Geometry: final body of the model. Coordinates: model frame, mm. Face numbers are marked on the shaded views. A direction names the side the tool comes from. Round coordinates to 2 decimals unless told otherwise and drop trailing zeros. Loops run counter-clockwise (first coordinate to the right, second up) from the corner with the lowest first, then second, coordinate; pieces in that order, holes last. Notation, with made-up numbers: M 0,-3.75 L 40,-3.75 A18 ccw 40,20.25 Z; hole C 5,-39.5 d3. An arc over 180 degrees is marked long. Answer as a JSON object with one key per item and string values.
from build123d import *

# Parameters (mm, degrees)
SKETCH_1_R          = 4.5
EXTRUDE_1_DEPTH     = 55
EXTRUDE_2_DEPTH     = 15
SKETCH_4_R          = 2
CUT_EXTRUDE_1_DEPTH = 71.544312315
CUT_EXTRUDE_3_DEPTH = 71.544312315
FILLET_1_R          = 0.5


with BuildPart() as part:
    # 草图1 → 凸台-拉伸1 (new body)
    with BuildSketch(Plane(origin=(0, 0, 0), x_dir=(1, 0, 0), z_dir=(0, 1, 0))):
        with Locations(Location((0, 0, 0), (0, 0, 270))):
            Circle(SKETCH_1_R)
    extrude(amount=EXTRUDE_1_DEPTH)

    # 草图2 → 凸台-拉伸2 (add)
    with BuildSketch(Plane(origin=(0, 55, 0), x_dir=(1, 0, 0), z_dir=(0, 1, 0))):
        with BuildLine():
            Line((-3, 3.010398645), (-3, -3.010398645))
            ThreePointArc((-3, -3.010398645), (0, -4.25), (3, -3.010398645))
            Line((3, -3.010398645), (3, 3.010398645))
            ThreePointArc((3, 3.010398645), (0, 4.25), (-3, 3.010398645))
        make_face()
    extrude(amount=EXTRUDE_2_DEPTH)

    # 草图4 → 切除-拉伸1 (cut, through all)
    with BuildSketch(Plane.ZY.offset(3)):
        with Locations((0, 61.5)):
            Circle(SKETCH_4_R)
    extrude(amount=-CUT_EXTRUDE_1_DEPTH, mode=Mode.SUBTRACT)

    # 草图5 → 切除-拉伸3 (cut, through all)
    with BuildSketch(Plane.ZY.offset(3)):
        with BuildLine():
            Line((-4.813255022, 64.251745482), (-4.813255022, 72.406434262))
            Line((-4.813255022, 72.406434262), (5.466876832, 72.406434262))
            Line((5.466876832, 72.406434262), (5.466876832, 63.634516306))
            ThreePointArc((5.466876832, 63.634516306), (0.449497866, 65.986517994), (-4.813255022, 64.251745482))
        make_face()
    extrude(amount=-CUT_EXTRUDE_3_DEPTH, mode=Mode.SUBTRACT)

    # 圆角1
    fillet_1_edges = [part.edges().sort_by_distance(p)[0] for p in [
        (0, 64.679603547, -4.25),
        (0, 64.679603547, 4.25),
    ]]
    fillet(fillet_1_edges, radius=FILLET_1_R)


solid = part.part
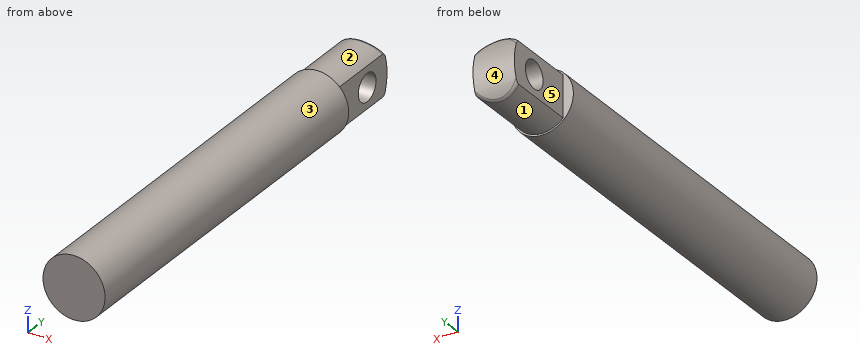
1) Ray query, line 1 (Y direction, x = -1.4, z = 0); line 2 (X direction, y = 60.5, z = -3.75); line 3 (X direction, y = 53, z = -2). Return the intervals inside material, ascending.
Results:
{"line 1": "0 to 59.5, 63.5 to 66", "line 2": "-2 to 2", "line 3": "-4.03 to 4.03"}
2) Section query A-A (z = 0). Return the cut outline in (x, y).
Results:
{"outline": "M -4.5,0 L 4.5,0 L 4.5,55 L 3,55 L 3,59.5 L -3,59.5 L -3,55 L -4.5,55 Z; M -3,63.5 L 3,63.5 L 3,66 L -3,66 Z"}
3) Reachability of the marked faces 1, 2, 3, 4 and 5 from +Z, -Z, +X, -X, +Y, -Y: full face, straight path, thin tool, end or side. Return the list, or none.
Results:
{"face 1": "-Z, +Y", "face 2": "+Z, +Y", "face 3": "+Y, -Y", "face 4": "+X, -X, +Y", "face 5": "+Z, -Z, -X, +Y"}
4) Section query C-C (y = 35.5). Return the cut outline in (x, z), and give its area (3 significant figures).
Results:
{"outline": "C 0,0 d9", "area": "63.6 mm2"}
5) Pin query (flat end, axial travel): P1, Ø5, axis at y = 61, z = 0.5, coming from the +X side; P2, Ø1, axis at y = 12, z = -1, coming from the +X side; P3, Ø4.5, axis at y = 61.5, z = 0, coming from the -X side; P4, Ø1.8, axis at y = 62, z = 0, coming from the -X side. Return the tip coordinate at first contact, or that it passes through.
Results:
{"P1": "x = 3", "P2": "x = 4.47", "P3": "x = -3", "P4": "through"}
6) Section query B-B (y = 61.5). Return the cut outline in (x, z), and give its area (3 significant figures).
Results:
{"outline": "M -3,-3.01 A4.25 ccw 3,-3.01 L 3,-2 L -3,-2 Z; M -3,2 L 3,2 L 3,3.01 A4.25 ccw -3,3.01 Z", "area": "22.4 mm2"}
